from build123d import *

# Parameters (mm, degrees)
INNER_START         = 1.5875
SKETCH1_R           = 1.143
INNER_LINK_S1_DEPTH = 0.762
TUBES_START         = 3.175
SKETCH3_R           = 1.651
SKETCH3_R_2         = 1.143
TUBES_DEPTH         = 3.175


with BuildPart() as part:
    # Sketch1 → inner link s1 (new body)
    with BuildSketch(Plane.XY.offset(INNER_START)):
        with BuildLine():
            ThreePointArc((-1.006284153, -2.769235484), (2.9464, 0), (-1.006284153, 2.769235484))
            ThreePointArc((-1.006284153, 2.769235484), (-3.175, 2.387415405), (-5.343715847, 2.769235484))
            ThreePointArc((-5.343715847, 2.769235484), (-9.2964, 0), (-5.343715847, -2.769235484))
            ThreePointArc((-5.343715847, -2.769235484), (-3.175, -2.387415405), (-1.006284153, -2.769235484))
        make_face()
        with Locations(Location((0, 0, 0), (0, 0, 180))):
            Circle(SKETCH1_R, mode=Mode.SUBTRACT)
        with Locations(Location((-6.35, 0, 0), (0, 0, 180))):
            Circle(SKETCH1_R, mode=Mode.SUBTRACT)
    extrude(amount=INNER_LINK_S1_DEPTH)


with BuildPart() as body_2:
    # inner link s2: mirrored copy
    add(part.part.mirror(Plane.XY))


with BuildPart() as part_1:
    add(part.part)

    add(body_2.part)  # tubes merges body 2
    # Sketch3 → tubes (add)
    # profile 1 of 2: a face of its own
    with BuildSketch(Plane(origin=(0, 0, 1.5875), x_dir=(-1, 0, 0), z_dir=(0, 0, -1)).offset(TUBES_START)):
        with Locations(Location((0, 0, 0), (0, 0, 180))):
            Circle(SKETCH3_R)
        Circle(SKETCH3_R_2, mode=Mode.SUBTRACT)
    # profile 2 of 2: a face of its own
    with BuildSketch(Plane(origin=(0, 0, 1.5875), x_dir=(-1, 0, 0), z_dir=(0, 0, -1)).offset(TUBES_START)):
        with Locations(Location((6.35, 0, 0), (0, 0, 180))):
            Circle(SKETCH3_R)
        with Locations((6.35, 0)):
            Circle(SKETCH3_R_2, mode=Mode.SUBTRACT)
    extrude(amount=-TUBES_DEPTH)


solid = part_1.part
Work out the finished part from the listing and answer in its coordinate system (mm). A direction names the side the tool comes from. Give positions to 0.01 mm unless a question says otherwise; leave off trailing zeros. Loops run counter-clockwise (first coordinate to the right, second up) from the corner with the lowest first, then second, coordinate; pieces in that order, holes last. Notation, with made-up numbers: (24, 63) - (78, 63) arc R16 ccw to (78, 91) - close; hole circle Ø3 at (58.5, 79). An arc over 180 degrees is marked (long way). Answer in a Markdown table with one row per item. Add a question column.
Q1. The part is cut by section B-B (y = 0). Determine the outline of the cut face in (x, z), and give its area (3 significant figures).
Q2. The part is cut by section A-A (x = -6.35). Determine the outline of the cut face in (y, z), and give its area (3 significant figures).
Q3. Each of these flat-tipped pins is pushed along its axis until it touches: P1, Ø1.5, axis at x = -6.5, z = -0.5, coming from the +Y side; P2, Ø1, axis at x = 1.5, z = 1, coming from the -Y side. Where does it stop, or does it pass through?
Q4. A tool of negligible diameter and unlimited length cuts with its end or side. For faces 1 (the cylindrical face through (-8, 0, 0)), 2 (the flat face through (-3, 0, 2.35)), from which of +Z, -Z, +X, -X, +Y, -Y can it reach the whole face along a straight path? Write none if from no direction.
Q5. Determine the mould class of faces 3 (the flat face through (-3, 0, 1.588)), 4 (the flat face through (-3, 0, -2.35)) for opening direction X: released by +X, released by -X, zero draft, split by the parting line, or undercut.
Q6. The part is cut by section D-D (y = 1.95). Determine the outline of the cut face in (x, z), and give its area (3 significant figures).
Q7. Consider line 1 along Z through (x, y) = (1, 1.45); line 2 along Y through (x, z) = (0, -1.8); line 3 along Y through (x, z) = (-6.35, 0.5). Determine where each line is inside the solid, lowest interval first.
Q8. The part is cut by section C-C (z = 1.45). Determine the outline of the cut face in (x, y).
Solution:
| question | item | result |
|---|---|---|
| 1 | outline | (-9.3, -2.35) - (-7.49, -2.35) - (-7.49, 2.35) - (-9.3, 2.35) - (-9.3, 1.59) - (-8, 1.59) - (-8, -1.59) - (-9.3, -1.59) - close; (-5.21, -2.35) - (-1.14, -2.35) - (-1.14, 2.35) - (-5.21, 2.35) - close; (1.14, -2.35) - (2.95, -2.35) - (2.95, -1.59) - (1.65, -1.59) - (1.65, 1.59) - (2.95, 1.59) - (2.95, 2.35) - (1.14, 2.35) - close; hole (-4.7, -1.59) - (-1.65, -1.59) - (-1.65, 1.59) - (-4.7, 1.59) - close |
| 1 | area | 18.1 mm² |
| 2 | outline | (-2.95, -2.35) - (-1.14, -2.35) - (-1.14, 2.35) - (-2.95, 2.35) - (-2.95, 1.59) - (-1.65, 1.59) - (-1.65, -1.59) - (-2.95, -1.59) - close; (1.14, -2.35) - (2.95, -2.35) - (2.95, -1.59) - (1.65, -1.59) - (1.65, 1.59) - (2.95, 1.59) - (2.95, 2.35) - (1.14, 2.35) - close |
| 2 | area | 8.72 mm² |
| 3 | P1 | stops at y = 1.65 |
| 3 | P2 | stops at y = -1.31 |
| 4 | face 1 | none |
| 4 | face 2 | +Z, +X, -X, +Y, -Y |
| 5 | face 3 | undercut |
| 5 | face 4 | zero draft |
| 6 | outline | (-8.56, -2.35) - (2.21, -2.35) - (2.21, -1.59) - (-8.56, -1.59) - close; (-8.56, 1.59) - (2.21, 1.59) - (2.21, 2.35) - (-8.56, 2.35) - close |
| 6 | area | 16.4 mm² |
| 7 | line 1 | z = -2.35 to -1.59, 1.59 to 2.35 |
| 7 | line 2 | y = -2.95 to -1.14, 1.14 to 2.95 |
| 7 | line 3 | y = -1.65 to -1.14, 1.14 to 1.65 |
| 8 | outline | circle Ø3.3 at (-6.35, 0); circle Ø3.3 at (0, 0); hole circle Ø2.29 at (-6.35, 0); hole circle Ø2.29 at (0, 0) |
